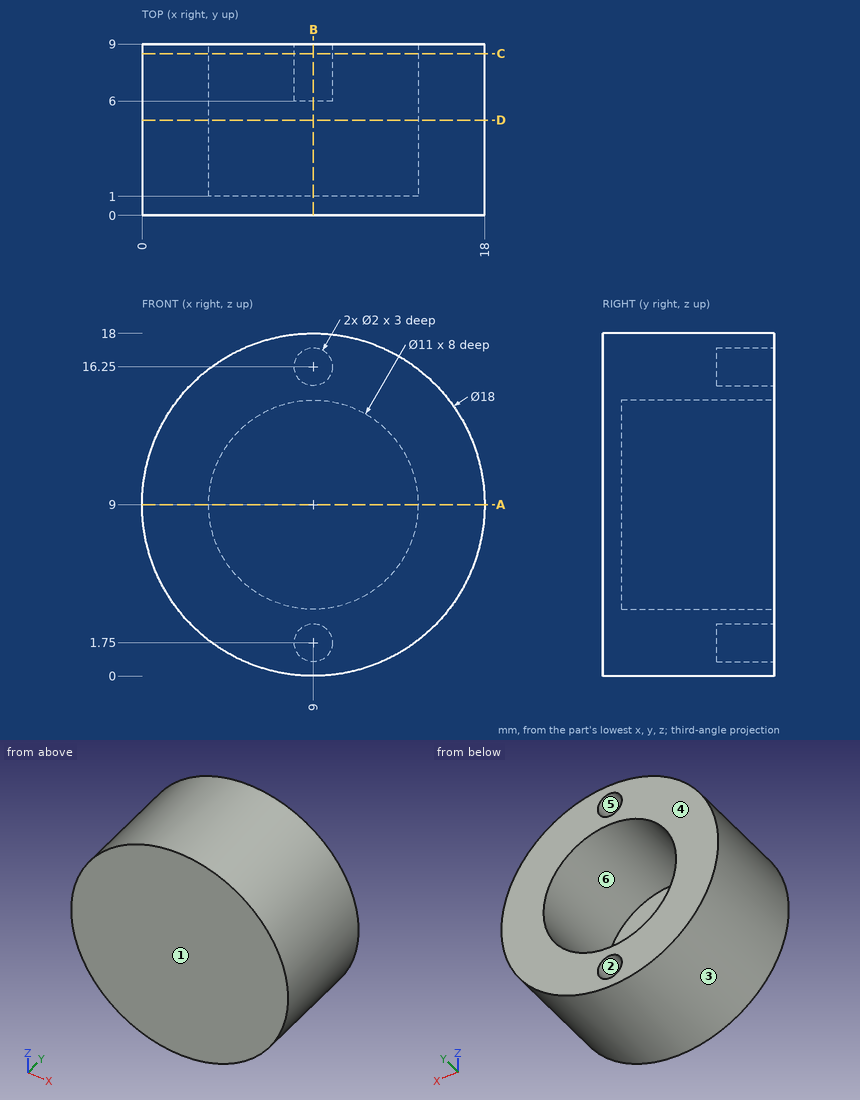
Part print with two shaded views. Sizes in mm from the minimum x, y, z corner. A direction names the side the tool comes from. Give positions to 0.01 mm unless a question says otherwise; leave off trailing zeros. Write each loop counter-clockwise with the first axis right and the second up, starting at its lowest first coordinate (ties: lowest second). Pieces come first, ordered by that corner, then holes.
1) Pin check, flat tips, straight feed: pin 1 (1.2 mm diameter, centred on x = 9, z = 16.25, fed in from -Y); pin 2 (9 mm diameter, centred on x = 9, z = 9, fed in from +Y); pin 3 (2 mm diameter, centred on x = 5.5, y = 1, fed in from +Z); pin 4 (1 mm diameter, centred on x = 7.5, y = 5.5, fed in from -Z). Stop position of each tip, or through.
Resolved:
pin 1: stops at y = 0
pin 2: stops at y = 1
pin 3: stops at z = 17.65
pin 4: stops at z = 0.06
2) Cut at D-D on y = 5. Write the cut outline in (x, z).
Resolved:
outline: circle Ø18 at (9, 9); hole circle Ø11 at (9, 9)
3) Probe L1, parallel to Z at x = 9, y = 7.75; L2, parallel to Z at x = 9, y = 3.5. List the from-to ranges inside material, lowest first.
Resolved:
L1: z = 0 to 0.75, 2.75 to 3.5, 14.5 to 15.25, 17.25 to 18
L2: z = 0 to 3.5, 14.5 to 18
4) Cut at B-B on x = 9. Write the cut outline in (y, z), then the cut area to 3 significant figures.
Resolved:
outline: (0, 0) - (9, 0) - (9, 0.75) - (6, 0.75) - (6, 2.75) - (9, 2.75) - (9, 3.5) - (1, 3.5) - (1, 14.5) - (9, 14.5) - (9, 15.25) - (6, 15.25) - (6, 17.25) - (9, 17.25) - (9, 18) - (0, 18) - close
area: 62.0 mm2
5) Cut at C-C on y = 8.5. Write the cut outline in (x, z), then the cut area to 3 significant figures.
Resolved:
outline: circle Ø18 at (9, 9); hole circle Ø11 at (9, 9); hole circle Ø2 at (9, 1.75); hole circle Ø2 at (9, 16.25)
area: 153 mm2
6) Two-plate mould, pull along X, no slides. Class the marked faces 3, 4, 5 and 6: released by +X, released by -X, zero draft, split by the parting line, or undercut.
Resolved:
face 3: split by the parting line
face 4: zero draft
face 5: undercut
face 6: undercut
7) Cut at A-A on z = 9. Write the cut outline in (x, y), then the cut area to 3 significant figures.
Resolved:
outline: (0, 0) - (18, 0) - (18, 9) - (14.5, 9) - (14.5, 1) - (3.5, 1) - (3.5, 9) - (0, 9) - close
area: 74.0 mm2
8) Which spindle directions (+Z, -Z, +X, -X, +Y, -Y) get a long thin tool onto all of the face, cutting with end or side? Do the marked faces 1 and 2. Say none if no direction does.
Resolved:
face 1: +Z, -Z, +X, -X, -Y
face 2: +Y
